from build123d import *

# Parameters (mm, degrees)
F0_W     = 125.034798
F0_H     = 113.135892
F1_DEPTH = 152.4
F3_DEPTH = 125.035798
F5_DEPTH = 125.035798
F6_R     = 28.062264
F7_DEPTH = 101.6
F8_R     = 21.423824
F9_DEPTH = 101.6


with BuildPart() as f1:
    # F0 (on Top) → F1 (new body)
    with BuildSketch(Plane.XY):
        with Locations((-2.346424, -0.839917)):
            Rectangle(F0_W, F0_H)
    extrude(amount=F1_DEPTH)

    # F2 (on face) → F3 (cut, through all)
    with BuildSketch(Plane.YZ.offset(60.170975)):
        Polygon((-57.407863, 152.4), (-57.407863, 0), (-33.916943, 152.4), align=None)
    extrude(amount=-F3_DEPTH, mode=Mode.SUBTRACT)

    # F4 (on face) → F5 (cut, through all)
    with BuildSketch(Plane.YZ.offset(60.170975)):
        Polygon((29.225653, 152.4), (55.728029, 0), (55.728029, 152.4), align=None)
    extrude(amount=-F5_DEPTH, mode=Mode.SUBTRACT)

    # F6 (on face) → F7 (join)
    with BuildSketch(Plane.XY.offset(152.4)):
        Circle(F6_R)
    extrude(amount=F7_DEPTH)

    # F8 (on face) → F9 (join)
    with BuildSketch(Plane.XY.offset(254)):
        Circle(F8_R)
    extrude(amount=F9_DEPTH)


solid = f1.part
The model under review builds one solid part; all positions refer to its coordinate system, in mm. A direction names the side the tool comes from. Coordinates: 2 decimals unless noted, no trailing zeros. Loops run counter-clockwise (first coordinate to the right, second up) from the corner with the lowest first, then second, coordinate; pieces in that order, holes last. Notation, with made-up numbers: M 24.25,16 L 33.25,16 A27 cw 33.25,49 Z; hole C -19.5,-13 d5. An arc over 180 degrees is marked long. Put each result on its own line as item: value. Start each with the question number.
Q1. The part is to be moulded in two halves that separate along Y. For faces 3 (the flat face through (-1.471, -45.827, 75.133)), 4 (the flat face through (-1.47, 42.29, 77.27)), 5 (the flat face through (-17, -23, 152.4)), 6 (the cylindrical face through (-6.083, -27.395, 202.489)), say which applies: +Y half, -Y half, draft (parallel to the pull), parting line (faces both ways), or undercut.
Q2. Wall thickness on line 1 (Z direction, x = 4.5, y = -26.5); line 2 (Z direction, x = 14.5, y = 24.5); line 3 (Y direction, x = 42.5, z = 92.5): over which ranges is each line inside the solid? List them lowest first.
Q3. Add section A-A (y = 0). Write out the cut boundary in (x, z).
Q4. Add section C-C (z = 218.5). Write out the cut boundary in (x, y), and give its area (3 significant figures).
Q5. Clearance check with flat-ended pins moving along their axes: pin 1 (2 mm diameter, centred on y = -19, z = 184.5, fed in from -X); pin 2 (8 mm diameter, centred on x = 39.5, z = 104.5, fed in from +Y); pin 3 (5 mm diameter, centred on x = 35.5, z = 110, fed in from -Y). State where each tip first meets the part, or that it passes through.
Q6. Add section B-B (x = 0). Write out the cut boundary in (y, z), and give its area (3 significant figures).
Q7. For faces 1 (the flat face through (-6, -21, 254)), 2 (the flat face through (-64.864, -2, 75)), list the 3-axis set-ups (+Z, -Z, +X, -X, +Y, -Y) from which the entire face can be reached by the end or side of a thin tool; tool diameter is ignored.
Q8. Add section D-D (x = -44). Write out the cut boundary in (y, z), and give its area (3 significant figures).
Answers:
1. face 3: -Y half
1. face 4: +Y half
1. face 5: draft
1. face 6: parting line
2. line 1: z = 0 to 254
2. line 2: z = 0 to 152.4
2. line 3: y = -43.15 to 39.64
3. outline: M -64.86,0 L 60.17,0 L 60.17,152.4 L 28.06,152.4 L 28.06,254 L 21.42,254 L 21.42,355.6 L -21.42,355.6 L -21.42,254 L -28.06,254 L -28.06,152.4 L -64.86,152.4 Z
4. outline: C 0,0 d56.12
4. area: 2,470 mm^2
5. pin 1: stops at x = -21.53
5. pin 2: stops at y = 38.25
5. pin 3: stops at y = -40.84
6. outline: M -57.41,0 L 55.73,0 L 29.23,152.4 L 28.06,152.4 L 28.06,254 L 21.42,254 L 21.42,355.6 L -21.42,355.6 L -21.42,254 L -28.06,254 L -28.06,152.4 L -33.92,152.4 Z
6. area: 23,500 mm^2
7. face 1: +Z
7. face 2: +Z, -Z, -X, +Y, -Y
8. outline: M -57.41,0 L 55.73,0 L 29.23,152.4 L -33.92,152.4 Z
8. area: 13,400 mm^2
